Design review of the part built by this model. Coordinates are the model's own, in mm. Face numbers are marked on the shaded views. A direction names the side the tool comes from. Coordinates: 2 decimals unless noted, no trailing zeros. Write each loop counter-clockwise with the first axis right and the second up, starting at its lowest first coordinate (ties: lowest second). Pieces come first, ordered by that corner, then holes.
Q1. Add section C-C, the plane y = 24. Give the boundary of the cut face in (x, z).
Q2. To check wall thickness, follow probe 1 along Z at (x, y) = (25.4, 36.5) (3 decimals); probe 2 along Z at (x, y) = (-8, 23); probe 3 along Y at (x, z) = (21, 50). State the ranges of each line that lie inside material, in increasing order.
Q3. Machinability: for the marked faces 1 and 2, which of the approach directions +Z, -Z, +X, -X, +Y, -Y give a long, thin tool a straight path to every point of the face, cutting with its end or side? Answer none if there is none.
Q4. Add section D-D, the plane z = 18. Give the boundary of the cut face in (x, y), plus the area to 3 significant figures.
Q5. The part is to be moulded in two halves that separate along Y. For the marked faces 3, 4 and 5, say which applies: +Y half, -Y half, draft (parallel to the pull), parting line (faces both ways), or undercut.
Q6. Add section A-A, the plane x = 25.4. Give the boundary of the cut face in (y, z) (3 decimals), plus the area to 3 significant figures.
Q7. Add section B-B, the plane z = 50.8. Give the boundary of the cut face in (x, y) (3 decimals), plus the area to 3 significant figures.
Q8. Clearance check with flat-ended pins moving along their axes: pin 1 Ø11.5 at (x, y) = (-34, 3.5) entering from +Z; pin 2 Ø1.5 at (x, y) = (44, 17) entering from +Z. State where each tip first meets the part, or that it passes through.
from build123d import *

# Parameters (mm, degrees)
F0_W      = 114.3
F0_H      = 63.5
F0_R      = 19.05
F1_DEPTH  = 12.7
F2_DEPTH  = 6.35
F3_W      = 6.35
F3_H      = 60.325
F4_DEPTH  = 50.8
F6_DEPTH  = 114.301
F7_W      = 101.6
F7_H      = 50.8
F7_R      = 3.175
F8_DEPTH  = 6.35
F9_R      = 3.17499
F11_DEPTH = 114.301


# Not quite as in the source:
# - a fillet or chamfer is up to 0.001 mm smaller than in the source, because OpenCascade refuses the exact size


with BuildPart() as f1:
    # F0 (on Top) → F1 (new body)
    with BuildSketch(Plane.XY):
        Rectangle(F0_W, F0_H)
        with Locations((-25.4, 0)):
            Circle(F0_R, mode=Mode.SUBTRACT)
        with Locations((25.4, 0)):
            Circle(F0_R, mode=Mode.SUBTRACT)
    extrude(amount=F1_DEPTH)

    # F0 (on Top) → F2 (join)
    with BuildSketch(Plane.XY):
        with Locations((-25.4, 0)):
            Circle(F0_R)
        with Locations((25.4, 0)):
            Circle(F0_R)
    extrude(amount=F2_DEPTH)

    # F3 (on face) → F4 (join)
    with BuildSketch(Plane.XY.offset(12.7)):
        with Locations((-53.975, 1.5875)):
            Rectangle(F3_W, F3_H)
        with Locations((53.975, 1.5875)):
            Rectangle(F3_W, F3_H)
    extrude(amount=F4_DEPTH)

    # F5 (on face) → F6 (cut, through all)
    with BuildSketch(Plane(origin=(-57.15, 0, 0), x_dir=(0, -1, 0), z_dir=(-1, 0, 0))):
        Polygon((28.575, 63.5), (-31.75, 63.5), (28.575, 12.7), align=None)
    extrude(amount=-F6_DEPTH, mode=Mode.SUBTRACT)

    # F7 (on face) → F8 (join)
    with BuildSketch(Plane(origin=(0, 31.75, 0), x_dir=(-1, 0, 0), z_dir=(0, 1, 0))):
        Polygon((-50.8, 12.7), (-50.8, 63.5), (-57.15, 63.5), (-57.15, 0), (57.15, 0), (57.15, 63.5), (50.8, 63.5), (50.8, 12.7), align=None)
        with Locations((0, 38.1)):
            Rectangle(F7_W, F7_H)
        with Locations((-25.4, 25.4)):
            Circle(F7_R, mode=Mode.SUBTRACT)
        with Locations((25.4, 25.4)):
            Circle(F7_R, mode=Mode.SUBTRACT)
        with Locations((-25.4, 50.8)):
            Circle(F7_R, mode=Mode.SUBTRACT)
        with Locations((25.4, 50.8)):
            Circle(F7_R, mode=Mode.SUBTRACT)
    extrude(amount=F8_DEPTH)

    # F9 (radius 3.175 in the source; OpenCascade refuses exactly that, so slightly less here)
    f9_edges = [f1.edges().sort_by_distance(p)[0] for p in [
        (-44.45, 0, 12.7),
        (6.35, 0, 12.7),
        (0, -31.75, 12.7),
        (57.15, -31.75, 6.35),
        (-57.15, -31.75, 6.35),
    ]]
    fillet(f9_edges, radius=F9_R)

    # F10 (on face) → F11 (cut, through all)
    with BuildSketch(Plane.YZ.offset(57.15)):
        Polygon((31.75, 12.7), (31.75, 57.15), (-18.8612597303, 12.7), align=None)
    extrude(amount=-F11_DEPTH, mode=Mode.SUBTRACT)


solid = f1.part
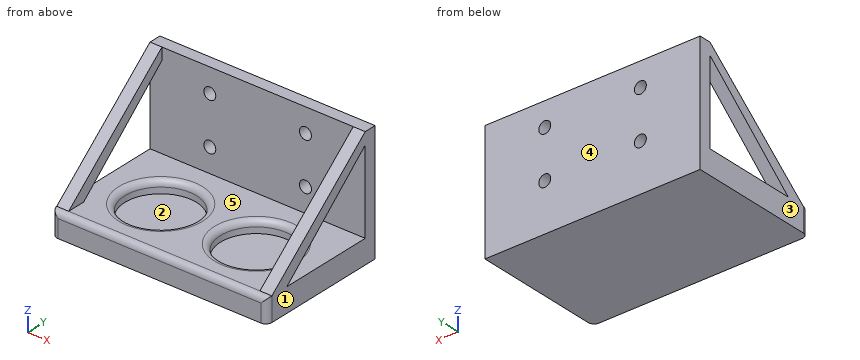
Here are the results:
1. outline: (-57.15, 0) - (57.15, 0) - (57.15, 12.7) - (-57.15, 12.7) - close; (-57.15, 50.34) - (-50.8, 50.34) - (-50.8, 56.97) - (-57.15, 56.97) - close; (50.8, 50.34) - (57.15, 50.34) - (57.15, 56.97) - (50.8, 56.97) - close
2. probe 1: z = 0 to 22.225, 28.575 to 47.625, 53.975 to 63.5
2. probe 2: z = 0 to 12.7
2. probe 3: y = 31.75 to 38.1
3. face 1: +Z, -Z, +X, +Y, -Y
3. face 2: +Z
4. outline: (-57.15, -22.28) - (-50.8, -22.28) - (-50.8, -12.83) - (-57.15, -12.83) - close; (-57.15, 31.75) - (57.15, 31.75) - (57.15, 38.1) - (-57.15, 38.1) - close; (50.8, -22.28) - (57.15, -22.28) - (57.15, -12.83) - (50.8, -12.83) - close
4. area: 846 mm2
5. face 3: draft
5. face 4: +Y half
5. face 5: undercut
6. outline: (-31.75, 0) - (38.1, 0) - (38.1, 22.225) - (31.75, 22.225) - (31.75, 12.7) - (22.225, 12.7) arc R3.175 ccw to (19.05, 9.525) - (19.05, 6.35) - (-19.05, 6.35) - (-19.05, 9.525) arc R3.175 ccw to (-22.225, 12.7) - (-28.575, 12.7) arc R3.175 ccw to (-31.75, 9.525) - close; (31.75, 28.575) - (38.1, 28.575) - (38.1, 47.625) - (31.75, 47.625) - close; (31.75, 53.975) - (38.1, 53.975) - (38.1, 63.5) - (31.75, 63.5) - close
6. area: 881 mm2
7. outline: (-57.15, 16.669) - (-50.8, 16.669) - (-50.8, 24.52) - (-57.15, 24.52) - close; (-57.15, 31.75) - (-28.575, 31.75) - (-28.575, 38.1) - (-57.15, 38.1) - close; (-22.225, 31.75) - (22.225, 31.75) - (22.225, 38.1) - (-22.225, 38.1) - close; (28.575, 31.75) - (57.15, 31.75) - (57.15, 38.1) - (28.575, 38.1) - close; (50.8, 16.669) - (57.15, 16.669) - (57.15, 24.52) - (50.8, 24.52) - close
7. area: 745 mm2
8. pin 1: stops at z = 6.35
8. pin 2: stops at z = 12.7
